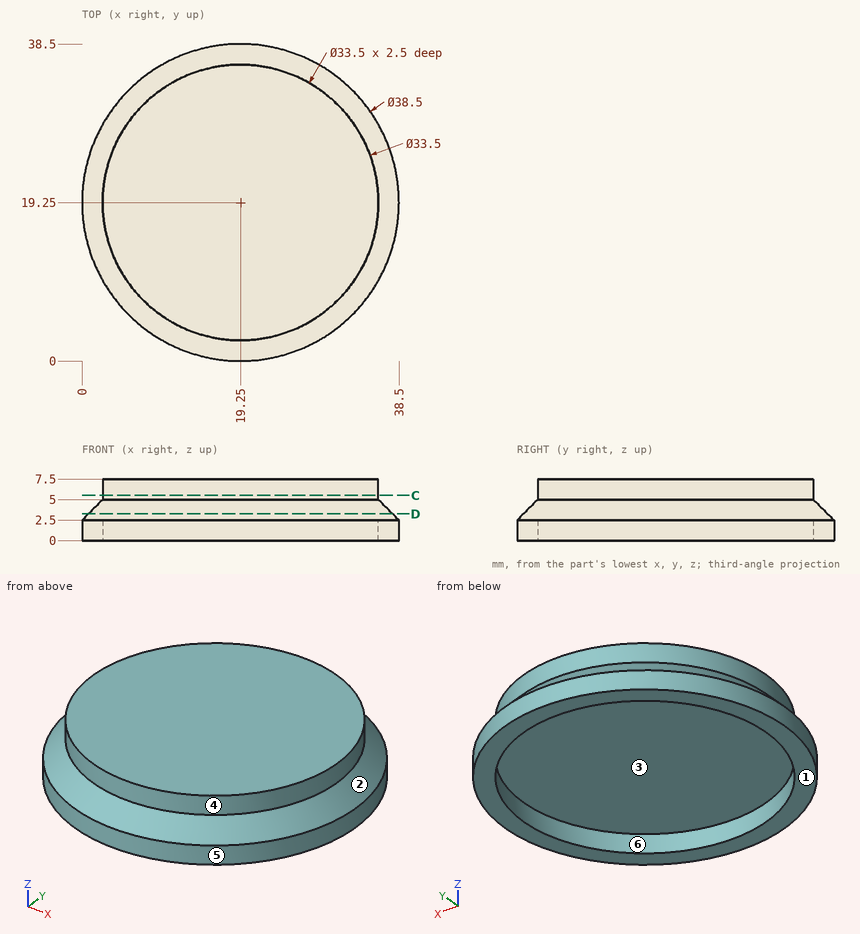
Check sheet for the drawn part. Datum: minimum x, y, z corner. Units: mm. A direction names the side the tool comes from. Coordinates: 2 decimals unless noted, no trailing zeros. Order: outer loops, then holes, each group sorted by start corner. A loop starts at its lowest first (then second) coordinate and runs counter-clockwise, first axis right, second up. Notation, with made-up numbers: (56, -28.75) - (101, -28.75) arc R18 ccw to (101, 6.25) - close; hole circle Ø1 at (19.25, 30). An arc over 180 degrees is marked (long way). Return JSON: item names as keys, results as strings.
(1) Go/stop test with flat-tipped pins: pin 1 (2 mm diameter, centred on x = 21.5, y = 21.5, fed in from -Z); pin 2 (1 mm diameter, centred on x = 30.5, z = 3.5, fed in from +Y); pin 3 (1 mm diameter, centred on x = 22.5, z = 1, fed in from +Y). Record where each tip stops, or that it passes through.
Filled sheet:
{"pin 1": "stops at z = 2.5", "pin 2": "stops at y = 34.35", "pin 3": "stops at y = 38.3"}
(2) Section check C-C, the plane z = 5.5. Record the cut outline in (x, y).
Filled sheet:
{"outline": "circle Ø33.5 at (19.25, 19.25)"}
(3) Access from +Z, -Z, +X, -X, +Y, -Y to the whole of each face (thin tool, end or side, straight path). Record for the marked faces 4, 5 and 6.
Filled sheet:
{"face 4": "+Z", "face 5": "+Z, -Z", "face 6": "-Z"}
(4) Section check D-D, the plane z = 3.25. Record the cut outline in (x, y).
Filled sheet:
{"outline": "circle Ø37 at (19.25, 19.25)"}
(5) Thickness scan on line 1 along Y through (x, z) = (19.25, 1.15); line 2 along Z through (x, y) = (25.5, 14); line 3 along Y through (x, z) = (28.5, 1.75). Record the ranges inside material, lowest first.
Filled sheet:
{"line 1": "y = 0 to 2.5, 36 to 38.5", "line 2": "z = 2.5 to 7.5", "line 3": "y = 2.37 to 5.29, 33.21 to 36.13"}
(6) Mould release check, pull along Y, two halves, no side actions. Record for the marked faces 1, 2 and 3: pulls with the +Y half, pulls with the -Y half, needs draft (parallel to the pull), parting line crosses it, or undercut.
Filled sheet:
{"face 1": "needs draft", "face 2": "parting line crosses it", "face 3": "undercut"}
